Part model, mm, in its own coordinate system. A direction names the side the tool comes from. Coordinates: 2 decimals unless noted, no trailing zeros. Write each loop counter-clockwise with the first axis right and the second up, starting at its lowest first coordinate (ties: lowest second). Pieces come first, ordered by that corner, then holes. Notation, with made-up numbers: (12, 25) -> (60, 25) arc R13 cw to (60, 47) -> close; hole circle Ø3 at (67, 46). An arc over 180 degrees is marked (long way). Write item = value, one per line.
from build123d import *

# Parameters (mm, degrees)
SKETCH_1_W      = 17.2
SKETCH_1_H      = 48
EXTRUDE_1_DEPTH = 5.6
SKETCH_2_W      = 20
SKETCH_2_H      = 15
EXTRUDE_2_DEPTH = 9


with BuildPart() as part:
    # 草图1 → 凸台-拉伸1 (new body)
    with BuildSketch(Plane(origin=(0, 0, 0), x_dir=(0, -1, 0), z_dir=(-1, 0, 0))):
        Rectangle(SKETCH_1_W, SKETCH_1_H)
    extrude(amount=-EXTRUDE_1_DEPTH)

    # 草图2 → 凸台-拉伸2 (add)
    with BuildSketch(Plane(origin=(5.6, 0, 0), x_dir=(0, 0, -1), z_dir=(1, 0, 0))):
        with Locations((-14, 0)):
            Rectangle(SKETCH_2_W, SKETCH_2_H)
    extrude(amount=EXTRUDE_2_DEPTH)


solid = part.part
Q1. Probe line 1 (X direction, y = 1.25, z = -4); line 2 (Z direction, x = 8, y = -4.5); line 3 (Y direction, x = 10, z = 16). List the from-to ranges inside material, lowest first. Write a range as from..to.
Model answer:
line_1 = 0..5.6
line_2 = 4..24
line_3 = -7.5..7.5
Q2. Saw through at C-C on x = 8.5. Give the cut face in (y, z).
Model answer:
outline = (-7.5, 4) -> (7.5, 4) -> (7.5, 24) -> (-7.5, 24) -> close
Q3. Saw through at B-B on z = 9. Give the cut face in (x, y), and give its area (3 significant figures).
Model answer:
outline = (0, -8.6) -> (5.6, -8.6) -> (5.6, -7.5) -> (14.6, -7.5) -> (14.6, 7.5) -> (5.6, 7.5) -> (5.6, 8.6) -> (0, 8.6) -> close
area = 231 mm²
Q4. Saw through at D-D on z = -10.5. Give the cut face in (x, y).
Model answer:
outline = (0, -8.6) -> (5.6, -8.6) -> (5.6, 8.6) -> (0, 8.6) -> close
Q5. Pin check, flat tips, straight feed: pin 1 (1 mm diameter, centred on x = 8.5, z = 14, fed in from +Y); pin 2 (2.5 mm diameter, centred on x = 9.5, z = 13, fed in from -Y). Stop position of each tip, or through.
Model answer:
pin_1 = 7.5
pin_2 = -7.5
Q6. Saw through at A-A on y = -2.25. Give the cut face in (x, z), and give its area (3 significant figures).
Model answer:
outline = (0, -24) -> (5.6, -24) -> (5.6, 4) -> (14.6, 4) -> (14.6, 24) -> (0, 24) -> close
area = 449 mm²
Q7. Which spindle directions (+Z, -Z, +X, -X, +Y, -Y) get a long thin tool onto all of the face, cutting with end or side? Do faces 1 (the face through (10, -7.5, 14)), 2 (the face through (10, 7.5, 14)), 3 (the face through (10, 0, 4)). Say none if no direction does.
Model answer:
face_1 = +Z, -Z, +X, -Y
face_2 = +Z, -Z, +X, +Y
face_3 = -Z, +X, +Y, -Y
